from build123d import *

# Parameters (mm, degrees)
F0_W       = 20
F0_H       = 20
F1_DEPTH   = 20
F2_R       = 5.4812551749
F1_FACE_W  = 20
F1_FACE_H  = 20
F3_DEPTH   = 20
F4_R       = 4.7702363178
F1_FACE2_W = 20
F1_FACE2_H = 20
F5_DEPTH   = 20
F6_R       = 7.6111370414
F7_DEPTH   = 20


with BuildPart() as f1:
    # F0 (on Top) → F1 (new body)
    with BuildSketch(Plane.XY):
        with Locations((10, 10)):
            Rectangle(F0_W, F0_H)
    extrude(amount=F1_DEPTH)

    # F2 (on Top) + F1_face (on face) → F3 (cut)
    with BuildSketch(Plane.XY):
        with Locations((9.7394008189, 10.2959359065)):
            Circle(F2_R)
    with BuildSketch(Plane(origin=(10, 10, 20), x_dir=(1, 0, 0), z_dir=(0, 0, 1))):
        Rectangle(F1_FACE_W, F1_FACE_H)
    extrude(amount=F3_DEPTH, mode=Mode.SUBTRACT)

    # F4 (on face) + F1_face2 (on face) → F5 (cut)
    with BuildSketch(Plane.YZ.offset(20)):
        with Locations((9.6540758386, 9.8292576149)):
            Circle(F4_R)
    with BuildSketch(Plane(origin=(0, 10, 10), x_dir=(0, -1, 0), z_dir=(-1, 0, 0))):
        Rectangle(F1_FACE2_W, F1_FACE2_H)
    extrude(amount=-F5_DEPTH, dir=(1, 0, 0), mode=Mode.SUBTRACT)

    # F6 (on face) → F7 (cut)
    with BuildSketch(Plane.XZ):
        with Locations((9.5273330808, 11.1748687923)):
            Circle(F6_R)
    extrude(amount=-F7_DEPTH, mode=Mode.SUBTRACT)


solid = f1.part
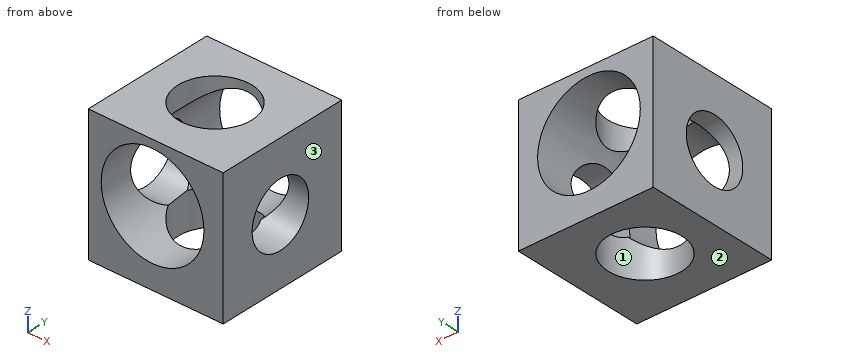
Work out the finished part from the listing and answer in its coordinate system (mm). Face numbers are marked on the shaded views. Give positions to 0.01 mm unless a question says otherwise; leave off trailing zeros. Loops run counter-clockwise (first coordinate to the right, second up) from the corner with the lowest first, then second, coordinate; pieces in that order, holes last. Notation, with made-up numbers: (54.25, 29.25) - (110.25, 29.25) arc R24 ccw to (110.25, 53.25) - close; hole circle Ø5 at (89, 44). An arc over 180 degrees is marked (long way). Answer in a Markdown table with one row per item.
(1) A flat-ended cylindrical pin translates along its axis: pin 1 Ø2 at (x, z) = (15, 14.5) entering from +Y. Find the tip coordinate at first contact, or state that the pin passes through.
Results list:
| item | result |
|---|---|
| pin 1 | passes through |
(2) Section A-A (x = 14.25) is taken. Give the vertices of the cut face in (y, z).
Results list:
| item | result |
|---|---|
| outline | (0, 0) - (7.18, 0) - (7.18, 5.21) - (0, 5.21) - close; (0, 17.14) - (7.18, 17.14) - (7.18, 20) - (0, 20) - close; (13.41, 0) - (20, 0) - (20, 5.21) - (13.41, 5.21) - close; (13.41, 17.14) - (20, 17.14) - (20, 20) - (13.41, 20) - close |
(3) Section D-D (y = 7.25) is taken. Give the vertices of the cut face in (x, z), and give its area (3 significant figures).
Results list:
| item | result |
|---|---|
| outline | (0, 0) - (5.18, 0) - (5.18, 4.93) arc R7.61 cw to (4.23, 5.71) - (0, 5.71) - close; (0, 13.95) - (2.44, 13.95) arc R7.61 cw to (5.18, 17.42) - (5.18, 20) - (0, 20) - close; (14.3, 0) - (20, 0) - (20, 5.71) - (14.82, 5.71) arc R7.61 cw to (14.3, 5.24) - close; (14.3, 17.11) arc R7.61 cw to (16.61, 13.95) - (20, 13.95) - (20, 20) - (14.3, 20) - close |
| area | 117 mm² |
(4) Section C-C (y = 15.5) is taken. Give the vertices of the cut face in (x, z), and give its area (3 significant figures).
Results list:
| item | result |
|---|---|
| outline | (0, 0) - (8.02, 0) - (8.02, 3.71) arc R7.61 cw to (8.02, 18.63) - (8.02, 20) - (0, 20) - close; (11.46, 0) - (20, 0) - (20, 20) - (11.46, 20) - (11.46, 18.54) arc R7.61 cw to (11.46, 3.81) - close |
| area | 201 mm² |
(5) Section B-B (z = 15.75) is taken. Give the vertices of the cut face in (x, y), and give its area (3 significant figures).
Results list:
| item | result |
|---|---|
| outline | (0, 0) - (3.44, 0) - (3.44, 20) - (0, 20) - close; (15.61, 0) - (20, 0) - (20, 20) - (15.61, 20) - close |
| area | 157 mm² |
(6) Consider L1, parallel to Y at x = 5, z = 1; L2, parallel to Y at x = 11.25, z = 19; L3, parallel to Z at x = 2.5, y = 4.5. Determine where each line is inside the solid, lowest interval first. Write a range as [from, to].
Results list:
| item | result |
|---|---|
| L1 | y = [0, 7.54], [13.05, 20] |
| L2 | y = [0, 5.03], [15.56, 20] |
| L3 | z = [0, 8.25], [14.1, 20] |
(7) For a pull along X with two mould halves and no side action, classify the marked faces 1, 2 and 3 as pulls with the +X half, pulls with the -X half, needs draft (parallel to the pull), parting line crosses it, or undercut.
Results list:
| item | result |
|---|---|
| face 1 | undercut |
| face 2 | needs draft |
| face 3 | pulls with the +X half |
